Here's the drawing with two shaded views (mm, measured from the low corner). I have some questions. A direction names the side the tool comes from. Coordinates: 2 decimals unless noted, no trailing zeros. Loops run counter-clockwise (first coordinate to the right, second up) from the corner with the lowest first, then second, coordinate; pieces in that order, holes last. Notation, with made-up numbers: (-4.5, 71) - (52.5, 71) arc R19 ccw to (52.5, 98) - close; hole circle Ø7 at (52.5, 75). An arc over 180 degrees is marked (long way). One line per item, written item: value. Start each with the question number.
(1) On a 3-axis mill with a long thin cutter (end or side, diameter ignored), from which of +Z, -Z, +X, -X, +Y, -Y can I reach the whole of each face in a straight line? I mean the marked faces 1 and 2. Say none if no direction works.
(2) If we section it at D-D on y = 13: Write out the boundary of the cut face in (x, z) (1 decimal), then the cut area to 3 significant figures.
(3) If I drill on line 1 along Y through (x, z) = (74, 17); line 2 along Z through (x, y) = (75, 2.5); line 3 along X through (y, z) = (10, 32.5) (1 decimal), over which ranges is the centre line in solid material (lowest first)? Write a range as from..to.
(4) If we section it at C-C on z = 24.5: Write out the boundary of the cut face in (x, y) (1 decimal).
(5) If we section it at A-A on y = 37: Write out the boundary of the cut face in (x, z) (1 decimal).
(6) If we section it at B-B on x = 35.5: Write out the boundary of the cut face in (y, z), then the cut area to 3 significant figures.
(7) I'm going to push a flat-ended pin straight in: P1, Ø3, axis at x = 58.5, y = 9.5, coming from the +Z side. Where does the tip first touch, or does it pass through?
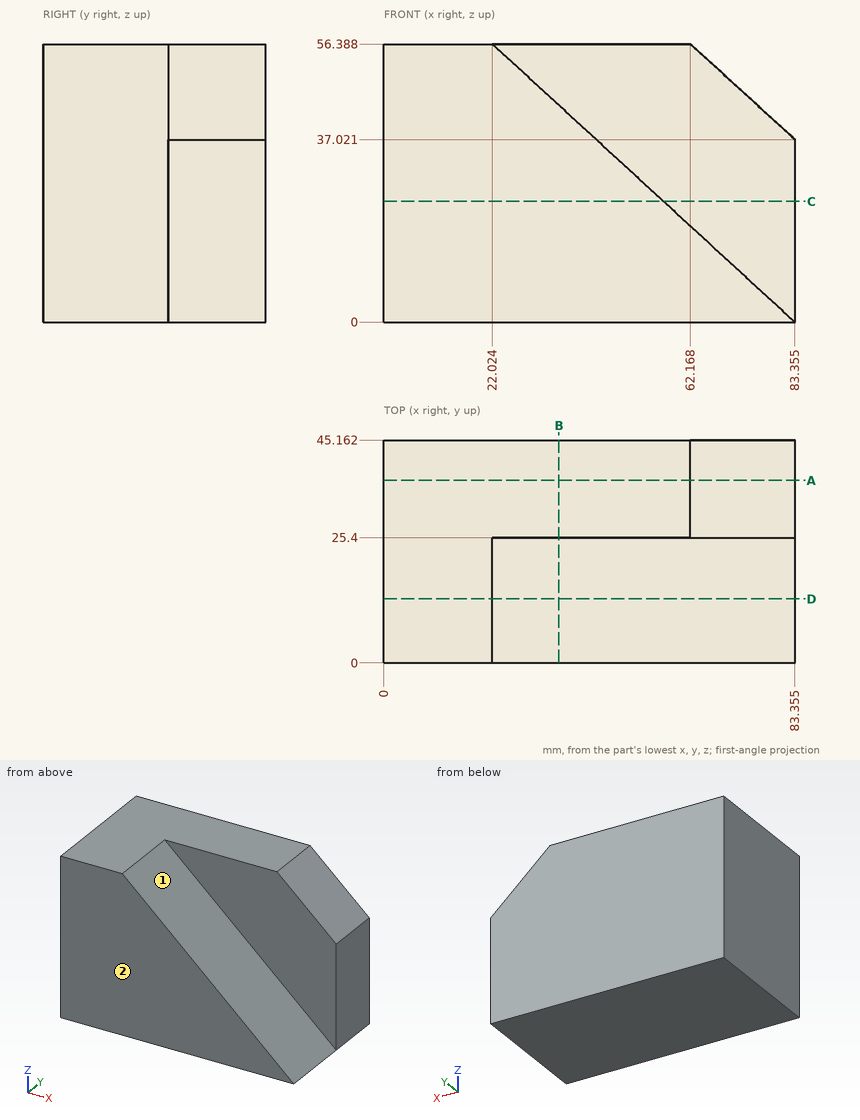
Values:
1. face 1: +Z, +X, -Y
1. face 2: +Z, -Z, +X, -X, -Y
2. outline: (0, 0) - (83.4, 0) - (22, 56.4) - (0, 56.4) - close
2. area: 2,970 mm2
3. line 1: y = 25.4..45.16
3. line 2: z = 0..7.68
3. line 3: x = 0..48
4. outline: (0, 0) - (56.7, 0) - (56.7, 25.4) - (83.4, 25.4) - (83.4, 45.2) - (0, 45.2) - close
5. outline: (0, 0) - (83.4, 0) - (83.4, 37) - (62.2, 56.4) - (0, 56.4) - close
6. outline: (0, 0) - (45.16, 0) - (45.16, 56.39) - (25.4, 56.39) - (25.4, 44) - (0, 44) - close
6. area: 2,230 mm2
7. P1: stops at z = 24.23
